Could you check a few things on this model? Use its own coordinates, in mm. A direction names the side the tool comes from. Give positions to 0.01 mm unless a question says otherwise; leave off trailing zeros. Put each result on its own line as item: value.
from build123d import *

# Parameters (mm, degrees)
BOSS_EXTRUDE1_DEPTH = 5
BOSS_EXTRUDE2_REACH = 84.916
SKETCH3_R           = 5
CUT_EXTRUDE1_DEPTH  = 25
SKETCH4_R           = 6.5
CUT_EXTRUDE2_DEPTH  = 3
FILLET1_R           = 1


with BuildPart() as part:
    # Sketch1 → Boss-Extrude1 (new body)
    with BuildSketch(Plane.XY):
        with BuildLine():
            Line((-16.204881352, 35), (-16.204881352, -35))
            Line((-16.204881352, -35), (66.332495807, -35))
            ThreePointArc((66.332495807, -35), (75, 0), (66.332495807, 35))
            Line((66.332495807, 35), (-16.204881352, 35))
        make_face()
    extrude(amount=BOSS_EXTRUDE1_DEPTH)

    # Boss-Extrude2: up to this plane
    boss_extrude2_end = Plane(origin=(7.525658293, -40, 47.009794297), z_dir=(-0.239863978039186, 0, -0.9708065059728519))
    # Sketch2 → Boss-Extrude2 (add, up to the surface)
    with BuildSketch(Plane.XY.offset(5), mode=Mode.PRIVATE) as boss_extrude2_sk1:
        with BuildLine():
            Line((65.295118648, 33.5), (-14.704881352, 33.5))
            Line((-14.704881352, 33.5), (-14.704881352, -33.5))
            Line((-14.704881352, -33.5), (65.295118648, -33.5))
            ThreePointArc((65.295118648, -33.5), (73.141235595, 0), (65.295118648, 33.5))
        make_face()
    boss_extrude2_tool1 = split(extrude(boss_extrude2_sk1.sketch, amount=BOSS_EXTRUDE2_REACH, mode=Mode.PRIVATE), bisect_by=boss_extrude2_end, keep=Keep.BOTH, mode=Mode.PRIVATE)
    add(boss_extrude2_tool1.solids().sort_by_distance((27.970522, 0, 5))[0])

    # Sketch3 → Cut-Extrude1 (cut)
    with BuildSketch(Plane(origin=(11.379758408, 0, 46.057534728), x_dir=(0.970806505972852, 0, -0.23986397803918558), z_dir=(0.2398639780391856, 0, 0.9708065059728521))):
        with Locations((-16.869040946, 25)):
            Circle(SKETCH3_R)
        with Locations((-16.869040946, -25)):
            Circle(SKETCH3_R)
        with Locations((48.130959054, -25)):
            Circle(SKETCH3_R)
        with Locations((48.130959054, 25)):
            Circle(SKETCH3_R)
    extrude(amount=-CUT_EXTRUDE1_DEPTH, mode=Mode.SUBTRACT)

    # Sketch4 → Cut-Extrude2 (cut)
    with BuildSketch(Plane(origin=(11.379758408, 0, 46.057534728), x_dir=(0.970806505972852, 0, -0.23986397803918558), z_dir=(0.2398639780391856, 0, 0.9708065059728521))):
        with Locations((-16.869040946, 25)):
            Circle(SKETCH4_R)
        with Locations((-16.869040946, -25)):
            Circle(SKETCH4_R)
        with Locations((48.130959054, -25)):
            Circle(SKETCH4_R)
        with Locations((48.130959054, 25)):
            Circle(SKETCH4_R)
    extrude(amount=-CUT_EXTRUDE2_DEPTH, mode=Mode.SUBTRACT)

    # Fillet1
    fillet1_edges = [part.edges().sort_by_distance(p)[0] for p in [
        (25.295118648, -33.5, 42.619368994),
        (-14.704881352, 0, 52.502449775),
        (25.295118648, 33.5, 42.619368994),
        (73.141235595, 0, 30.797693023),
        (-11.307058581, 25, 51.662925852),
        (51.795364307, 25, 36.07176728),
        (51.795364307, -25, 36.07176728),
        (-11.307058581, -25, 51.662925852),
    ]]
    fillet(fillet1_edges, radius=FILLET1_R - 0.0001)  # a hair under: the kernel refuses the full size


solid = part.part
1) Which directions (+Z, -Z, +X, -X, +Y, -Y) give clear straight access to the entire face, cutting with the end or side of a thin tool? Please do faces 1 (the cylindrical face through (73.14, -0.49, 18.27)), 2 (the flat face through (-7.62, -29.78, 47.66)), 3 (the cylindrical face through (24.918, -33.215, 42.403)).
Filled in:
face 1: +Z, +X
face 2: none
face 3: +Z, +X, -Y
2) I'm going to push flat-ended pins straight in: pin 1 (1 mm diameter, centred on x = 40, y = 6, fed in from +Z); pin 2 (6 mm diameter, centred on x = 26.5, z = 44, fed in from +Y); pin 3 (23 mm diameter, centred on x = 6.5, z = 18, fed in from -Y). Where does each tip first touch, or does it pass through?
Filled in:
pin 1: stops at z = 39.11
pin 2: stops at y = 33.5
pin 3: stops at y = -33.5
3) We'd pull the mould along Z, two halves only. Please class faces 4 (the flat face through (22, 34, 5)), 5 (the cylindrical face through (-3.834, -26.915, 35.554)), 6 (the flat face through (-14.705, 0, 28)), 7 (the cylindrical face through (53.73, -29.88, 21.33)): pulls with the +Z half, pulls with the -Z half, needs draft (parallel to the pull), parting line crosses it, or undercut.
Filled in:
face 4: pulls with the +Z half
face 5: undercut
face 6: needs draft
face 7: undercut
4) Suppose I cut it at A-A, the plane z = 19.5. State how many separate pieces and enclosed holes the cut face has, and give its area (3 significant figures).
Filled in:
separate pieces: 1
enclosed holes: 2
area: 5,550 mm^2
5) If I drill on line 1 (Y direction, x = 20.5, z = 20); line 2 (Y direction, x = 67, z = 28.5); line 3 (Z direction, x = 44.5, y = 18), over which ranges is the centre line in solid material (lowest first)? Write a range as [from, to].
Filled in:
line 1: y = [-33.5, 33.5]
line 2: y = [-29.81, 29.81]
line 3: z = [0, 37.87]
